For this review, take the finished solid that the model builds, in its own axes (mm). A direction names the side the tool comes from. Coordinates: 2 decimals unless noted, no trailing zeros. Order: outer loops, then holes, each group sorted by start corner. A loop starts at its lowest first (then second) coordinate and runs counter-clockwise, first axis right, second up. Notation, with made-up numbers: (52.25, -21) -> (86.25, -21) arc R12 ccw to (86.25, -14) -> close; hole circle Ø6 at (50, -26.75). An arc over 180 degrees is marked (long way). Answer as a JSON object with one key per item and string values. Group by question number.
1) Draft analysis for pull direction Y (two halves, no side actions). For faces 1 (the cylindrical face through (24, -14.95, -0.81)), 2 (the flat face through (-22, -12, 2.5)), 3 (the cylindrical face through (23.95, 15, -0.81)), 4 (the cylindrical face through (20.42, 13.68, -0.81)), state which applies: +Y half, -Y half, draft (parallel to the pull), parting line (faces both ways), or undercut.
2) Add section B-B, the plane z = 2. Write out the cut boundary in (x, y), then the cut area to 3 significant figures.
3) Wall thickness on L1, parallel to Y at x = 21.5, z = -0.95; L2, parallel to X at y = -12.5, z = -0.8; L3, parallel to X at y = -10.5, z = 4.75: over which ranges is each line inside the solid? List them lowest first.
4) Machinability: for faces 5 (the flat face through (0, 16, 2)), 6 (the flat face through (-19, 10, 0)), which of the approach directions +Z, -Z, +X, -X, +Y, -Y give a long, thin tool a straight path to every point of the face, cutting with its end or side? Answer none if there is none.
5) For pin 1 (2 mm diameter, centred on y = -11, z = 2.5, fed in from +X); pin 2 (3 mm diameter, centred on x = 20, y = 11.5, fed in from +Z); pin 3 (4 mm diameter, centred on y = 9.5, z = 3, fed in from +X), all flat-tipped, find the tip position at first contact; note any pin that passes through.
6) Add section C-C, the plane y = 8. Write out the cut boundary in (x, z).
7) Add section A-A, the plane z = -1. Write out the cut boundary in (x, y), then the cut area to 3 significant figures.
Autodesk Inventor part; units mm, degrees
ref_plane "YZ Plane" through (0, 0, 0) normal (1, 0, 0) x (0, 1, 0)
ref_plane "XZ Plane" through (0, 0, 0) normal (0, 1, 0) x (-1, 0, 0)
ref_plane "XY Plane" through (0, 0, 0) normal (0, 0, 1) x (1, 0, 0)
sketch "Sketch1" plane through (0, 0, 0) normal (0, 0, 1) x (1, 0, 0)
  line L0 (25, 16) -> (-25, 16)
  line L1 (-25, 16) -> (-25, -16)
  line L2 (-25, -16) -> (25, -16)
  line L3 (25, -16) -> (25, 16)
  line L4 (25, 16) -> (-25, -16) construction
  line L5 (-25, 16) -> (25, -16) construction
  line L6 (0, 16) -> (0, -16) construction
  line L7 (25, 0) -> (-25, 0) construction
  line L8 (0, -16) -> (0, 16) construction
  line L9 (21.5, -12.5) -> (21.5, 12.5) construction
  circle A0 centre (-21.5, -12.5) radius 3
  circle A1 centre (-21.5, 12.5) radius 3
  arc A2 (-19.5635, -16) -> (-25, -10.5635) centre (-21.5, -12.5) ccw
  arc A3 (-25, 10.5635) -> (-19.5635, 16) centre (-21.5, 12.5) ccw
  arc A4 (25, -10.5635) -> (19.5635, -16) centre (21.5, -12.5) ccw
  arc A5 (19.5635, 16) -> (25, 10.5635) centre (21.5, 12.5) ccw
  point P0 (0, 0)
  point P1 (21.5, 0)
  point P2 (25, 10.5635)
  point P3 (19.5635, 16)
  point P4 (-19.5635, 16)
  point P5 (-25, 10.5635)
  point P6 (19.5635, -16)
  point P7 (25, -10.5635)
  dimension "d0" = 50
  dimension "d1" = 32
  dimension "d18" = 3.5
  dimension "d19" = 25
  dimension "d21" = 6
  dimension "d24" = 1
extrude "Extrusion1" add sketch "Sketch1" against normal blind 1.6 contours L3 A5 L0 | A5 L3 A4 L2 A2 L1 A3 L0 | A3 L1 L0 | L3 L2 A4 | A2 L2 L1 | A0 | A1
extrude "Extrusion2" add sketch "Sketch1" along normal blind 2.5 contours A0 | A1
hole "Phi3.2" at (21.5, -12.5, 0) at (21.5, 12.5, 0) direction (0, 0, -1) diameter 3.2 end through all
fillet "R3.5" radius 3.5 4 edges at (25, -16, -0.8) (-25, -16, -0.8) (-25, 16, -0.8) (25, 16, -0.8)
extrude "Extrusion3" add sketch "Sketch1" along normal blind 5.5 contours A5 L3 A4 L2 A2 L1 A3 L0
fillet "R2" radius 2 8 edges at (19.5635, -16, 2.75) (25, -10.5635, 2.75) (25, 10.5635, 2.75) (19.5635, 16, 2.75) (-19.5635, -16, 2.75) (-25, -10.5635, 2.75) (-25, 10.5635, 2.75) (-19.5635, 16, 2.75)
equation "\"d18\" = -0.5 * d19 + 0.5 * d1"
properties part number "SEN0539-EN" material "CFRP"
Output values:
{
 "1": {"face 1": "-Y half", "face 2": "draft", "face 3": "+Y half", "face 4": "undercut"},
 "2": {"outline": "(-25, -6.69) arc R2 ccw to (-22.5, -8.63) arc R4 cw to (-17.63, -13.5) arc R2 ccw to (-15.69, -16) -> (15.69, -16) arc R2 ccw to (17.63, -13.5) arc R4 cw to (22.5, -8.63) arc R2 ccw to (25, -6.69) -> (25, 6.69) arc R2 ccw to (22.5, 8.63) arc R4 cw to (17.63, 13.5) arc R2 ccw to (15.69, 16) -> (-15.69, 16) arc R2 ccw to (-17.63, 13.5) arc R4 cw to (-22.5, 8.63) arc R2 ccw to (-25, 6.69) -> close; circle Ø6 at (-21.5, -12.5); circle Ø6 at (-21.5, 12.5)", "area": "1,440 mm²"},
 "3": {"L1": "y = -16 to -14.1, -10.9 to 10.9, 14.1 to 16", "L2": "x = -25 to 19.9, 23.1 to 25", "L3": "x = -18.04 to 18.04"},
 "4": {"face 5": "+Z, -Z, +X, -X, +Y", "face 6": "+Z"},
 "5": {"pin 1": "stops at x = 18.38", "pin 2": "stops at z = 0", "pin 3": "stops at x = 24.83"},
 "6": {"outline": "(-25, -1.6) -> (25, -1.6) -> (25, 0) -> (24.51, 0) -> (24.51, 5.5) -> (-24.51, 5.5) -> (-24.51, 0) -> (-25, 0) -> close"},
 "7": {"outline": "(-25, -12.5) arc R3.5 ccw to (-21.5, -16) -> (21.5, -16) arc R3.5 ccw to (25, -12.5) -> (25, 12.5) arc R3.5 ccw to (21.5, 16) -> (-21.5, 16) arc R3.5 ccw to (-25, 12.5) -> close; hole circle Ø3.2 at (21.5, -12.5); hole circle Ø3.2 at (21.5, 12.5)", "area": "1,570 mm²"}
}
